Geometry check sheet. Reference: the model listing, model coordinates, mm. A direction names the side the tool comes from. Give positions to 0.01 mm unless a question says otherwise; leave off trailing zeros. Order: outer loops, then holes, each group sorted by start corner. A loop starts at its lowest first (then second) coordinate and runs counter-clockwise, first axis right, second up.
```python
from build123d import *

# Parameters (mm, degrees)
SKETCH_1_W           = 50
SKETCH_1_H           = 40
EXTRUDE_1_DEPTH      = 4
SKETCH_2_R           = 2
CUT_EXTRUDE_1_DEPTH  = 4
EXTRUDE_2_DEPTH      = 180
CUT_EXTRUDE_START    = -60
CUT_EXTRUDE_2_DEPTH  = 60
CUT_EXTRUDE_3_DEPTH  = 60
EXTRUDE_3_REACH      = 191.95
EXTRUDE_3_END_RADIUS = 230
EXTRUDE_START        = 38
EXTRUDE_4_DEPTH      = 38
CUT_EXTRUDE_4_DEPTH  = 211.154705038
SKETCH_9_R           = 3.5
EXTRUDE_5_DEPTH      = 40
SKETCH_10_R          = 1.5
CUT_EXTRUDE_5_DEPTH  = 30
CHAMFER_1_SIZE       = 0.5
EXTRUDE_6_REACH      = 171.111
EXTRUDE_6_END_RADIUS = 235
EXTRUDE_7_REACH      = 171.111
FILLET_1_R           = 10


with BuildPart() as part:
    # 草图1 → 凸台-拉伸1 (new body)
    with BuildSketch(Plane(origin=(0, 0, 0), x_dir=(0, 0, -1), z_dir=(1, 0, 0))):
        with Locations((0, -20)):
            Rectangle(SKETCH_1_W, SKETCH_1_H)
    extrude(amount=EXTRUDE_1_DEPTH)

    # 草图2 → 切除-拉伸1 (cut)
    with BuildSketch(Plane(origin=(4, 0, 0), x_dir=(0, 0, -1), z_dir=(1, 0, 0))):
        with Locations((-15, -10)):
            Circle(SKETCH_2_R)
        with Locations((15, -10)):
            Circle(SKETCH_2_R)
    extrude(amount=-CUT_EXTRUDE_1_DEPTH, mode=Mode.SUBTRACT)

    # 草图3 → 凸台-拉伸2 (add)
    with BuildSketch(Plane(origin=(4, 0, 0), x_dir=(0, 0, -1), z_dir=(1, 0, 0))):
        with BuildLine():
            Line((-25, -33.637267303), (-25, -38.666428911))
            ThreePointArc((-25, -38.666428911), (0, -40), (25, -38.666428911))
            Line((25, -38.666428911), (25, -33.637267303))
            ThreePointArc((25, -33.637267303), (0, -35), (-25, -33.637267303))
        make_face()
    extrude(amount=EXTRUDE_2_DEPTH)

    # 草图4 → 切除-拉伸2 (cut)
    with BuildSketch(Plane(origin=(4, 0, 0), x_dir=(0, 0, -1), z_dir=(1, 0, 0)).offset(CUT_EXTRUDE_START)):
        with BuildLine():
            Line((25, -40), (25, -38.666428911))
            ThreePointArc((25, -38.666428911), (12.517771485, -39.666370401), (0, -40))
            Line((0, -40), (25, -40))
        make_face()
    extrude(amount=CUT_EXTRUDE_2_DEPTH, mode=Mode.SUBTRACT)

    # 草图5 → 切除-拉伸3 (cut)
    with BuildSketch(Plane(origin=(4, 0, 0), x_dir=(0, 0, -1), z_dir=(1, 0, 0)).offset(CUT_EXTRUDE_START)):
        with BuildLine():
            Line((-25, -38.666428911), (-25, -40))
            Line((-25, -40), (0, -40))
            ThreePointArc((0, -40), (-12.517771485, -39.666370401), (-25, -38.666428911))
        make_face()
    extrude(amount=CUT_EXTRUDE_3_DEPTH, mode=Mode.SUBTRACT)

    # 凸台-拉伸3: up to this cylinder (the profile starts outside it)
    extrude_3_end = Plane(origin=(65.000728, 195, 0), z_dir=(-1, 0, 0)) * Cylinder(EXTRUDE_3_END_RADIUS, 844.9, mode=Mode.PRIVATE)
    # 草图6 → 凸台-拉伸3 (add, up to the surface)
    with BuildSketch(Plane(origin=(0, -40, 0), x_dir=(-1, 0, 0), z_dir=(0, -1, 0)), mode=Mode.PRIVATE) as extrude_3_sk1:
        with BuildLine():
            Line((-85.002334196, 61.845829501), (-85.002334196, 25))
            Line((-85.002334196, 25), (-125, 25))
            ThreePointArc((-125, 25), (-130, 0), (-125, -25))
            Line((-125, -25), (-85.002334196, -25))
            Line((-85.002334196, -25), (-85.002334196, -61.845829501))
            ThreePointArc((-85.002334196, -61.845829501), (-65.002453212, -64.999999954), (-45.002334196, -61.84733917))
            Line((-45.002334196, -61.84733917), (-45.002334196, -25))
            Line((-45.002334196, -25), (-5, -25))
            ThreePointArc((-5, -25), (0, 0), (-5, 25))
            Line((-5, 25), (-45.002334196, 25))
            Line((-45.002334196, 25), (-45.002334196, 61.84733917))
            ThreePointArc((-45.002334196, 61.84733917), (-65.002453212, 64.999999954), (-85.002334196, 61.845829501))
        make_face()
    extrude_3_tool1 = extrude(extrude_3_sk1.sketch, amount=-EXTRUDE_3_REACH, mode=Mode.PRIVATE) - extrude_3_end
    extrude_3 = extrude_3_tool1.solids().sort_by_distance((65.000728, -40, 0))[0]
    add(extrude_3)

    # 镜向1: 凸台-拉伸3 across plane
    add(extrude_3.mirror(Plane.XY))

    # 草图7 → 凸台-拉伸4 (add)
    with BuildSketch(Plane.XZ.offset(40).offset(EXTRUDE_START)):
        with BuildLine():
            Line((5, -25), (8.810588186, -25))
            ThreePointArc((8.810588186, -25), (3.5, 0), (8.810588186, 25))
            Line((8.810588186, 25), (5, 25))
            ThreePointArc((5, 25), (1.26225608, 12.747548784), (0, 0))
            ThreePointArc((0, 0), (1.26225608, -12.747548784), (5, -25))
        make_face()
        with BuildLine():
            Line((45.002334196, -58.157917452), (45.002334196, -61.84733917))
            ThreePointArc((45.002334196, -61.84733917), (65.002453212, -64.999999954), (85.002334196, -61.845829501))
            Line((85.002334196, -61.845829501), (85.002334196, -58.156312011))
            ThreePointArc((85.002334196, -58.156312011), (65.002468367, -61.49999995), (45.002334196, -58.157917452))
        make_face()
        with BuildLine():
            Line((121.189411814, -25), (125, -25))
            ThreePointArc((125, -25), (128.73774392, -12.747548784), (130, 0))
            ThreePointArc((130, 0), (128.73774392, 12.747548784), (125, 25))
            Line((125, 25), (121.189411814, 25))
            ThreePointArc((121.189411814, 25), (126.5, 0), (121.189411814, -25))
        make_face()
        with BuildLine():
            Line((85.002334196, 58.156312011), (85.002334196, 61.845829501))
            ThreePointArc((85.002334196, 61.845829501), (65.002453212, 64.999999954), (45.002334196, 61.84733917))
            Line((45.002334196, 61.84733917), (45.002334196, 58.157917452))
            ThreePointArc((45.002334196, 58.157917452), (65.002468367, 61.49999995), (85.002334196, 58.156312011))
        make_face()
    extrude(amount=-EXTRUDE_4_DEPTH)

    # 草图8 → 切除-拉伸4 (cut, through all)
    with BuildSketch(Plane.XZ.offset(78)):
        with BuildLine():
            Line((184, 25), (125, 25))
            ThreePointArc((125, 25), (130, 0), (125, -25))
            Line((125, -25), (184, -25))
            Line((184, -25), (184, 25))
        make_face()
    extrude(amount=-CUT_EXTRUDE_4_DEPTH, mode=Mode.SUBTRACT)

    # 草图9 → 凸台-拉伸5 (add)
    with BuildSketch(Plane.XZ.offset(78)):
        with Locations((130, 0)):
            Circle(SKETCH_9_R)
        with Locations((65.002453212, -64.999999954)):
            Circle(SKETCH_9_R)
        with Locations((65.002453212, 64.999999954)):
            Circle(SKETCH_9_R)
    extrude(amount=-EXTRUDE_5_DEPTH)

    # 草图10 → 切除-拉伸5 (cut)
    with BuildSketch(Plane.XZ.offset(78)):
        with Locations(Location((65.002453212, 64.999999954, 0), (0, 0, 270))):
            Circle(SKETCH_10_R)
        with Locations(Location((130, 0, 0), (0, 0, 270))):
            Circle(SKETCH_10_R)
        with Locations(Location((65.002453212, -64.999999954, 0), (0, 0, 270))):
            Circle(SKETCH_10_R)
    extrude(amount=-CUT_EXTRUDE_5_DEPTH, mode=Mode.SUBTRACT)

    # 倒角1
    chamfer_1_edges = [part.edges().sort_by_distance(p)[0] for p in [
        (65.002453212, -78, 66.499999954),
        (130, -78, 1.5),
        (65.002453212, -78, -63.499999954),
    ]]
    chamfer(chamfer_1_edges, length=CHAMFER_1_SIZE)

    # 凸台-拉伸6: up to this cylinder (the profile starts outside it)
    extrude_6_end = Plane(origin=(1.489564, 195, 0), z_dir=(-1, 0, 0)) * Cylinder(EXTRUDE_6_END_RADIUS, 813.222, mode=Mode.PRIVATE)
    # 草图11 → 凸台-拉伸6 (add, up to the surface)
    with BuildSketch(Plane.XZ.offset(78), mode=Mode.PRIVATE) as extrude_6_sk1:
        with BuildLine():
            Line((0, 25), (0, 0))
            ThreePointArc((0, 0), (1.26225608, 12.747548784), (5, 25))
            Line((5, 25), (0, 25))
        make_face()
    extrude_6_tool1 = extrude(extrude_6_sk1.sketch, amount=-EXTRUDE_6_REACH, mode=Mode.PRIVATE) - extrude_6_end
    add(extrude_6_tool1.solids().sort_by_distance((1.489564, -78, 18.799089))[0])

    # 草图12 → 凸台-拉伸7 (add, up to next)
    with BuildSketch(Plane.XZ.offset(78), mode=Mode.PRIVATE) as extrude_7_sk1:
        with BuildLine():
            Line((0, -25), (5, -25))
            ThreePointArc((5, -25), (1.26225608, -12.747548784), (0, 0))
            Line((0, 0), (0, -25))
        make_face()
    extrude_7_tool1 = extrude(extrude_7_sk1.sketch, amount=-EXTRUDE_7_REACH, mode=Mode.PRIVATE) - part.part
    add(extrude_7_tool1.solids().sort_by_distance((1.489564, -78, -18.799089))[0])

    # 圆角1
    fillet_1_edges = [part.edges().sort_by_distance(p)[0] for p in [
        (2, 0, 25),
        (2, 0, -25),
    ]]
    fillet(fillet_1_edges, radius=FILLET_1_R)


solid = part.part
```
Q1. Cross-section at A-A, the plane y = -55. Record the boundary of the cut face in (x, z), and give its area (3 significant figures).
Q2. Gauge pin test, flat ends, axial feed: P1, Ø2.5, axis at x = 65, z = 65, coming from the +Y side; P2, Ø2, axis at x = 53, y = -41, coming from the +Z side; P3, Ø1.5, axis at x = 129.5, z = 0, coming from the -Y side. Record the tip position at first contact, or that the pin passes through.
Q3. Release check for a two-part mould opening along Z. For faces 1 (the face through (12, -39, -25)), 2 (the face through (85.002, -39, 50)), 3 (the face through (3.5, -59.3, -0.4)) record: pulls with the +Z half, pulls with the -Z half, needs draft (parallel to the pull), parting line crosses it, or undercut.
Q4. Cross-section at B-B, the plane z = -7.5. Record the boundary of the cut face in (x, y).
Q5. Cross-section at D-D, the plane y = -6. Record the boundary of the cut face in (x, z), and give its area (3 significant figures).
Q6. Thickness scan on L1, parallel to Z at x = 130, y = -61.5; L2, parallel to X at y = -32.5, z = 19; L3, parallel to X at y = -68, z = -65. Record the ranges inside material, lowest first.
Q7. Cross-section at C-C, the plane x = 50. Record the boundary of the cut face in (y, z), and give its area (3 significant figures).
Q8. Access from +Z, -Z, +X, -X, +Y, -Y to the whole of each face (thin tool, end or side, straight path). Record for faces 4 (the face through (45.002, -39, 49)), 5 (the face through (45.002, -39, -50)), 6 (the face through (64.7, -59.3, 61.5)).
Answers follow:
1. outline: (0, -25) - (8.81, -25) arc R61.5 cw to (8.81, 25) - (0, 25) - close; (45, -61.85) arc R65 ccw to (61.5, -64.91) arc R3.5 ccw (long way) to (68.5, -64.91) arc R65 ccw to (85, -61.85) - (85, -58.16) arc R61.5 cw to (45, -58.16) - close; (45, 58.16) arc R61.5 cw to (85, 58.16) - (85, 61.85) arc R65 ccw to (68.5, 64.91) arc R3.5 ccw (long way) to (61.5, 64.91) arc R65 ccw to (45, 61.85) - close; (121.19, -25) - (125, -25) arc R65 ccw to (129.91, -3.5) arc R3.5 ccw (long way) to (129.91, 3.5) arc R65 ccw to (125, 25) - (121.19, 25) arc R61.5 cw to start; hole circle Ø3 at (65, -65); hole circle Ø3 at (65, 65); hole circle Ø3 at (130, 0)
1. area: 764 mm2
2. P1: stops at y = -25.62
2. P2: stops at z = 64.06
2. P3: stops at y = -48
3. face 1: pulls with the -Z half
3. face 2: needs draft
3. face 3: undercut
4. outline: (0, -78) - (3.96, -78) - (3.96, -40) - (126.04, -40) - (126.04, -78) - (129.57, -78) - (129.57, -34.88) - (4, -34.88) - (4, 0) - (0, 0) - close
5. outline: (0, -24.17) - (4, -24.17) - (4, 24.17) - (0, 24.17) - close
5. area: 193 mm2
6. L1: z = -3.5 to -1.5, 1.5 to 3.5
6. L2: x = 0 to 4
6. L3: x = 61.5 to 63.5, 66.5 to 68.5
7. outline: (-78, -63.25) - (-26.13, -63.25) arc R230 cw to (-26.13, 63.25) - (-78, 63.25) - (-78, 59.64) - (-40, 59.64) - (-40, -59.64) - (-78, -59.64) - close
7. area: 1,280 mm2
8. face 4: +Z, -X, +Y, -Y
8. face 5: -Z, -X, +Y, -Y
8. face 6: -Y
